Geometry check sheet. Reference: the model listing, model coordinates, mm. A direction names the side the tool comes from. Coordinates: 2 decimals unless noted, no trailing zeros. Order: outer loops, then holes, each group sorted by start corner. A loop starts at its lowest first (then second) coordinate and runs counter-clockwise, first axis right, second up. Notation, with made-up numbers: (-25, 8.25) - (-11, 8.25) arc R5 ccw to (-11, 17.25) - close; hole circle Ø4 at (-35, 53). An arc over 180 degrees is marked (long way). One line per item, written item: value. Start each with the question number.
```python
from build123d import *

# Parameters (mm, degrees)
BOSS_EXTRUDE1_DEPTH    = 5.5
CUT_EXTRUDE1_DEPTH     = 3.5
FILLET2_R              = 4
SKETCH19_R             = 1.4
CUT_EXTRUDE3_DEPTH     = 6.3
SKETCH21_R             = 2.4
CUT_EXTRUDE4_DEPTH     = 4.5
BOSS_EXTRUDE3_DEPTH    = 1.3
FILLET5_R              = 0.3
FILLET6_R              = 1
BOSS_EXTRUDE4_DEPTH    = 5.5
SKETCH13_R             = 0.5
CUT_EXTRUDE5_DEPTH     = 6.5
FILLET7_R              = 0.1
SKETCH30_W             = 41.665308381
SKETCH30_H             = 8.97901041
CUT_EXTRUDE6_DEPTH     = 0.15
SKETCH31_W             = 41.594909832
SKETCH31_H             = 8.905627214
CUT_EXTRUDE7_DEPTH     = 0.15
M1_6_CLEARANCE_HOLE1_D = 1.7
CUT_EXTRUDE8_DEPTH     = 4.5


with BuildPart() as part:
    # Sketch1 → Boss-Extrude1 (new body)
    with BuildSketch(Plane(origin=(0, 0, 0), x_dir=(1, 0, 0), z_dir=(0, 1, 0))):
        Polygon((0, 0), (38, 0), (30, -8), (0, -8), align=None)
    extrude(amount=BOSS_EXTRUDE1_DEPTH)

    # Sketch4 → Cut-Extrude1 (cut)
    with BuildSketch(Plane.XY.offset(8)):
        Polygon((0, 0.5), (6, 0.5), (6, 0), (38, 0), (38, 5.5), (6, 5.5), (6, 5), (0, 5), align=None)
    extrude(amount=-CUT_EXTRUDE1_DEPTH, mode=Mode.SUBTRACT)

    # Fillet2
    fillet2_edges = [part.edges().sort_by_distance(p)[0] for p in [
        (0, 5.25, 8),
        (0, 2.75, 0),
    ]]
    fillet(fillet2_edges, radius=FILLET2_R - 0.0001)  # a hair under: the kernel refuses the full size

    # Sketch19 → Cut-Extrude3 (cut)
    with BuildSketch(Plane(origin=(0, 5.5, 0), x_dir=(1, 0, 0), z_dir=(0, 1, 0))):
        with Locations(Location((4, -4, 0), (0, 0, 270))):
            Circle(SKETCH19_R)
    extrude(amount=-CUT_EXTRUDE3_DEPTH, mode=Mode.SUBTRACT)

    # Sketch21 → Cut-Extrude4 (cut)
    with BuildSketch(Plane(origin=(0, 0.5, 0), x_dir=(1, 0, 0), z_dir=(0, 1, 0))):
        with Locations((4, -4)):
            Circle(SKETCH21_R)
    extrude(amount=CUT_EXTRUDE4_DEPTH, mode=Mode.SUBTRACT)

    # Sketch22 → Boss-Extrude3 (add)
    with BuildSketch(Plane.XY.offset(4.5)):
        Polygon((6.347338919, 5), (6, 5), (6, 5.5), (33.5, 5.5), (33.5, 0), (6, 0), (6, 0.5), (6.347338919, 0.5), align=None)
    extrude(amount=BOSS_EXTRUDE3_DEPTH)

    # Fillet5
    fillet5_edges = [part.edges().sort_by_distance(p)[0] for p in [
        (6, 0.25, 5.8),
        (6, 5.25, 5.8),
    ]]
    fillet(fillet5_edges, radius=FILLET5_R)

    # Fillet6
    fillet6_edges = [part.edges().sort_by_distance(p)[0] for p in [
        (6, 5.25, 8),
        (6, 0.25, 8),
    ]]
    fillet(fillet6_edges, radius=FILLET6_R)

    # Sketch25 → Boss-Extrude4 (add)
    with BuildSketch(Plane(origin=(0, 5.5, 0), x_dir=(1, 0, 0), z_dir=(0, 1, 0))):
        Polygon((38, 0), (33.5, -4.5), (33.5, -5.8), (34.646204889, -5.8), align=None)
    extrude(amount=-BOSS_EXTRUDE4_DEPTH)

    # Sketch13 → Cut-Extrude5 (cut)
    with BuildSketch(Plane(origin=(0, 0, 0), x_dir=(-1, 0, 0), z_dir=(0, 0, -1))):
        with Locations((-33.84, 4.25)):
            Circle(SKETCH13_R)
        with Locations((-33.84, 1.75)):
            Circle(SKETCH13_R)
    extrude(amount=-CUT_EXTRUDE5_DEPTH, mode=Mode.SUBTRACT)

    # Fillet7
    fillet7_edges = [part.edges().sort_by_distance(p)[0] for p in [
        (38, 2.75, 0),
    ]]
    fillet(fillet7_edges, radius=FILLET7_R)

    # Sketch30 → Cut-Extrude6 (cut)
    with BuildSketch(Plane(origin=(0, 5.5, 0), x_dir=(1, 0, 0), z_dir=(0, 1, 0))):
        with Locations((19.118021654, -4.03845395)):
            Rectangle(SKETCH30_W, SKETCH30_H)
    extrude(amount=-CUT_EXTRUDE6_DEPTH, mode=Mode.SUBTRACT)

    # Sketch31 → Cut-Extrude7 (cut)
    with BuildSketch(Plane(origin=(0, 0, 0), x_dir=(-1, 0, 0), z_dir=(0, -1, 0))):
        with Locations((-18.959670937, -4.021529517)):
            Rectangle(SKETCH31_W, SKETCH31_H)
    extrude(amount=-CUT_EXTRUDE7_DEPTH, mode=Mode.SUBTRACT)

    # M1.6 Clearance Hole1 (through all)
    with Locations(Plane(origin=(0, 0, 0), x_dir=(-1, 0, 0), z_dir=(0, 0, -1))):
        with Locations((-16, 2.75), (-28, 2.75)):
            Hole(M1_6_CLEARANCE_HOLE1_D / 2)

    # Sketch37 → Cut-Extrude8 (cut)
    with BuildSketch(Plane.XZ.offset(-5)):
        with BuildLine():
            Line((4, -0.442176814), (4, 8.442176814))
            ThreePointArc((4, 8.442176814), (-0.442176814, 4), (4, -0.442176814))
        make_face()
    extrude(amount=CUT_EXTRUDE8_DEPTH, mode=Mode.SUBTRACT)


solid = part.part
```
Q1. Gauge pin test, flat ends, axial feed: P1, Ø0.5, axis at y = 2.5, z = 0.5, coming from the -X side; P2, Ø1.5, axis at y = 3.5, z = 5, coming from the -X side; P3, Ø2.5, axis at x = 4, z = 4, coming from the +Y side. Record the tip position at first contact, or that the pin passes through.
Q2. Cross-section at D-D, the plane x = 28. Enter the section's corners in (y, z), and give its area (3 significant figures).
Q3. Release check for a two-part mould opening along Y. For faces 1 (the flat face through (2, 0.5, 4)), 2 (the flat face through (20, 3, 5.8)), 3 (the flat face through (19, 5.35, 3)), 4 (the cylindrical face through (34.34, 1.77, 2.86)) record: released by +Y, released by -Y, zero draft, split by the parting line, or undercut.
Q4. Set-up check for faces 5 (the flat face through (4, 3, 1)), 6 (the flat face through (6.347, 3, 5)), 7 (the cylindrical face through (5.88, 2.72, 2.51)): record each of +Z, -Z, +X, -X, +Y, -Y from which the full face is reachable in a straight line by a thin tool's end or side.
Q5. Cross-section at A-A, the plane y = 2.75. Enter the section's corners in (x, z), and give its area (3 significant figures).
Q6. Material ranges on probe 1 along Y at (x, z) = (33.84, 2.7); probe 2 along Y at (x, z) = (28, 2.25); probe 3 along X at (y, z) = (2.8, 2), recorded low to high.
Q7. Cross-section at C-C, the plane y = 4.25. Enter the section's corners in (x, z).
Q8. Cross-section at B-B, the plane x = 33.84. Enter the section's corners in (y, z), and give its area (3 significant figures).
Check result:
1. P1: stops at x = 4
1. P2: stops at x = 6.35
1. P3: passes through
2. outline: (0.15, 0) - (1.9, 0) - (1.9, 5.8) - (0.15, 5.8) - close; (3.6, 0) - (5.35, 0) - (5.35, 5.8) - (3.6, 5.8) - close
2. area: 20.3 mm2
3. face 1: undercut
3. face 2: zero draft
3. face 3: released by +Y
3. face 4: undercut
4. face 5: +Z, -Z, -X
4. face 6: +Z, -X
4. face 7: -X
5. outline: (4, 0) - (15.15, 0) - (15.15, 5.8) - (6.35, 5.8) - (6.35, 4.5) arc R2.4 cw to (4, 1.6) - close; (16.85, 0) - (27.15, 0) - (27.15, 5.8) - (16.85, 5.8) - close; (28.85, 0) - (37.83, 0) arc R0.1 ccw to (37.91, 0.15) - (34.65, 5.8) - (28.85, 5.8) - close
5. area: 159 mm2
6. probe 1: y = 0.15 to 1.25, 2.25 to 3.75, 4.75 to 5.35
6. probe 2: y = 0.15 to 1.9, 3.6 to 5.35
6. probe 3: x = 5.33 to 15.15, 16.85 to 27.15, 28.85 to 36.84
7. outline: (4, 0) - (33.34, 0) - (33.34, 5.8) - (6.35, 5.8) - (6.35, 4.5) arc R2.4 cw to (4, 1.6) - close; (34.34, 0) - (37.83, 0) arc R0.1 ccw to (37.91, 0.15) - (34.65, 5.8) - (34.34, 5.8) - close
8. outline: (0.15, 0) - (1.25, 0) - (1.25, 5.8) - (0.15, 5.8) - close; (2.25, 0) - (3.75, 0) - (3.75, 5.8) - (2.25, 5.8) - close; (4.75, 0) - (5.35, 0) - (5.35, 5.8) - (4.75, 5.8) - close
8. area: 18.6 mm2
